Geometry check sheet. Reference: the model listing, model coordinates, mm. Coordinates: 2 decimals unless noted, no trailing zeros. Loops run counter-clockwise (first coordinate to the right, second up) from the corner with the lowest first, then second, coordinate; pieces in that order, holes last. Notation, with made-up numbers: (-11.5, 58.25) - (44.5, 58.25) arc R9 ccw to (44.5, 75.25) - close; hole circle Ø7 at (12, 62.25). An arc over 180 degrees is marked (long way). One line per item, written item: value.
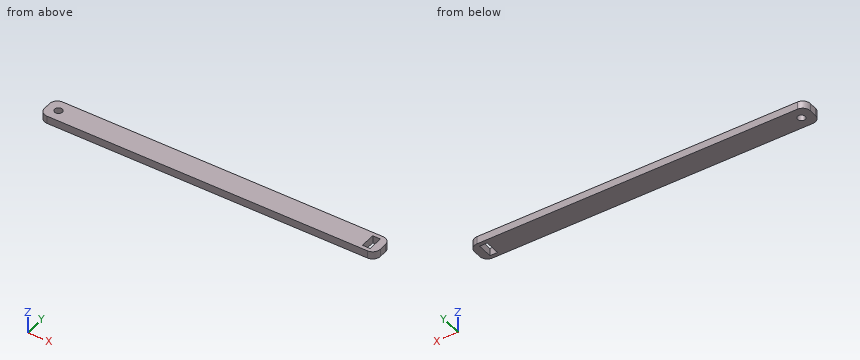
from build123d import *

# Parameters (mm, degrees)
SKETCH1_R           = 2.5
SKETCH1_W           = 5
SKETCH1_H           = 10
BOSS_EXTRUDE1_DEPTH = 5


with BuildPart() as part:
    # Sketch1 → Boss-Extrude1 (new body)
    with BuildSketch(Plane.XY):
        with BuildLine():
            Line((-215, 15), (-5, 15))
            ThreePointArc((-5, 15), (-1.464466094, 13.535533906), (0, 10))
            Line((0, 10), (0, 5))
            ThreePointArc((0, 5), (-1.464466094, 1.464466094), (-5, 0))
            Line((-5, 0), (-215, 0))
            ThreePointArc((-215, 0), (-218.535533906, 1.464466094), (-220, 5))
            Line((-220, 5), (-220, 10))
            ThreePointArc((-220, 10), (-218.535533906, 13.535533906), (-215, 15))
        make_face()
        with Locations((-212.5, 7.5)):
            Circle(SKETCH1_R, mode=Mode.SUBTRACT)
        with Locations((-7.5, 7.5)):
            Rectangle(SKETCH1_W, SKETCH1_H, mode=Mode.SUBTRACT)
    extrude(amount=BOSS_EXTRUDE1_DEPTH)


solid = part.part
(1) Go/stop test with flat-tipped pins: pin 1 Ø4 at (x, y) = (-212.5, 7.5) entering from +Z; pin 2 Ø1.5 at (y, z) = (2, 1) entering from +X. Record where each tip stops, or that it passes through.
Reply:
pin 1: through
pin 2: x = -0.53
(2) Cross-section at B-B on x = -212.5. Record the cut outline in (y, z).
Reply:
outline: (0, 0) - (5, 0) - (5, 5) - (0, 5) - close; (10, 0) - (15, 0) - (15, 5) - (10, 5) - close
(3) Cross-section at A-A on y = 7.5. Record the cut outline in (x, z).
Reply:
outline: (-220, 0) - (-215, 0) - (-215, 5) - (-220, 5) - close; (-210, 0) - (-10, 0) - (-10, 5) - (-210, 5) - close; (-5, 0) - (0, 0) - (0, 5) - (-5, 5) - close
(4) Cross-section at C-C on z = 3.1. Record the cut outline in (x, y).
Reply:
outline: (-220, 5) arc R5 ccw to (-215, 0) - (-5, 0) arc R5 ccw to (0, 5) - (0, 10) arc R5 ccw to (-5, 15) - (-215, 15) arc R5 ccw to (-220, 10) - close; hole circle Ø5 at (-212.5, 7.5); hole (-10, 2.5) - (-5, 2.5) - (-5, 12.5) - (-10, 12.5) - close
(5) Material ranges on probe 1 along X at (y, z) = (9.5, 4.75); probe 2 along X at (y, z) = (4.75, 0.4); probe 3 along Y at (x, z) = (-212.5, 3.85), recorded low to high. Write a range as from..to.
Reply:
probe 1: -220..-214, -211..-10, -5..0
probe 2: -219.99..-10, -5..-0.01
probe 3: 0..5, 10..15
